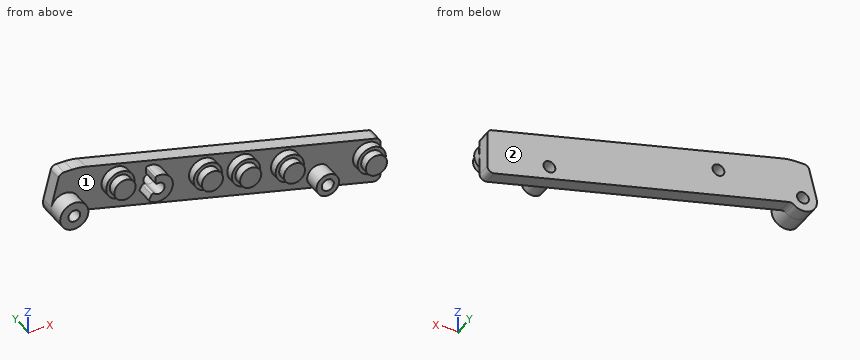
from build123d import *

# Parameters (mm, degrees)
SKETCH1_R           = 2.667
BOSS_EXTRUDE1_DEPTH = 6.35
SKETCH3_R           = 6.35
BOSS_EXTRUDE2_DEPTH = 3.81
SKETCH4_R           = 4.7625
BOSS_EXTRUDE3_DEPTH = 3.81
SKETCH5_R           = 6.35
SKETCH5_R_2         = 2.667
SKETCH5_R_3         = 5.08
SKETCH5_R_4         = 2.723974981
BOSS_EXTRUDE4_DEPTH = 7.62


with BuildPart() as part:
    # Sketch1 → Boss-Extrude1 (new body)
    with BuildSketch(Plane(origin=(0, 0, 0), x_dir=(-1, 0, 0), z_dir=(0, 1, 0))):
        with BuildLine():
            Line((132.859114436, 54.06756661), (1.925518385, 21.422154602))
            ThreePointArc((1.925518385, 21.422154602), (0.538452686, 20.521383604), (0, 18.957603457))
            Line((0, 18.957603457), (0, 3.251051746))
            ThreePointArc((0, 3.251051746), (0.976219853, 1.249504432), (3.154481615, 0.786500601))
            Line((3.154481615, 0.786500601), (135.868185597, 33.875743365))
            ThreePointArc((135.868185597, 33.875743365), (137.061865325, 33.884273202), (138.127619437, 33.346581632))
            ThreePointArc((138.127619437, 33.346581632), (145.587943549, 32.789337046), (148.401377862, 39.7212592))
            Line((148.401377862, 39.7212592), (145.116412217, 52.896536778))
            ThreePointArc((145.116412217, 52.896536778), (144.215641219, 54.283602477), (142.651861072, 54.822055163))
            Line((142.651861072, 54.822055163), (139.003930584, 54.822055163))
            ThreePointArc((139.003930584, 54.822055163), (135.908449262, 54.632727414), (132.859114436, 54.06756661))
        make_face()
        with Locations(Location((142.24, 38.185055163, 0), (0, 0, 90))):
            Circle(SKETCH1_R, mode=Mode.SUBTRACT)
        with Locations(Location((27.94, 12.785055202, 0), (0, 0, 90))):
            Circle(SKETCH1_R, mode=Mode.SUBTRACT)
        with Locations(Location((104.14, 38.185055202, 0), (0, 0, 90))):
            Circle(SKETCH1_R, mode=Mode.SUBTRACT)
    extrude(amount=-BOSS_EXTRUDE1_DEPTH)

    # Sketch3 → Boss-Extrude2 (add)
    with BuildSketch(Plane(origin=(0, -6.35, 0), x_dir=(-1, 0, 0), z_dir=(0, -1, 0))):
        with Locations(Location((6.00871488, -14.586933973, 0), (0, 0, 198.870092131))):
            Circle(SKETCH3_R)
        with Locations(Location((42.976982051, -23.804158196, 0), (0, 0, 270))):
            Circle(SKETCH3_R)
        with Locations(Location((79.945249222, -33.021382418, 0), (0, 0, 270))):
            Circle(SKETCH3_R)
        with Locations(Location((119.378067538, -42.853088255, 0), (0, 0, 270))):
            Circle(SKETCH3_R)
        with Locations(Location((62.693391209, -28.720011114, 0), (0, 0, 270))):
            Circle(SKETCH3_R)
    extrude(amount=BOSS_EXTRUDE2_DEPTH)

    # Sketch4 → Boss-Extrude3 (add)
    with BuildSketch(Plane.XZ.offset(10.16)):
        with Locations(Location((-6.00871488, 14.586933973, 0), (0, 0, 90))):
            Circle(SKETCH4_R)
        with Locations(Location((-42.976982051, 23.804158196, 0), (0, 0, 90))):
            Circle(SKETCH4_R)
        with Locations(Location((-62.693391209, 28.720011114, 0), (0, 0, 90))):
            Circle(SKETCH4_R)
        with Locations(Location((-79.945249222, 33.021382418, 0), (0, 0, 90))):
            Circle(SKETCH4_R)
        with Locations(Location((-119.378067538, 42.853088255, 0), (0, 0, 90))):
            Circle(SKETCH4_R)
    extrude(amount=BOSS_EXTRUDE3_DEPTH)

    # Sketch5 → Boss-Extrude4 (add)
    with BuildSketch(Plane.XZ.offset(6.35)):
        with Locations(Location((-142.24, 38.185055163, 0), (0, 0, 166))):
            Circle(SKETCH5_R)
        with Locations(Location((-142.24, 38.185055163, 0), (0, 0, 90))):
            Circle(SKETCH5_R_2, mode=Mode.SUBTRACT)
        with Locations(Location((-27.94, 12.785055202, 0), (0, 0, 270))):
            Circle(SKETCH5_R_3)
        with Locations(Location((-27.94, 12.785055202, 0), (0, 0, 270))):
            Circle(SKETCH5_R_4, mode=Mode.SUBTRACT)
        with BuildLine():
            Line((-105.580163175, 43.777970545), (-105.715311414, 41.562252701))
            ThreePointArc((-105.715311414, 41.562252701), (-105.443232026, 40.931048752), (-104.773674962, 40.775681582))
            ThreePointArc((-104.773674962, 40.775681582), (-101.589970205, 37.403878498), (-106.115998075, 36.393876649))
            ThreePointArc((-106.115998075, 36.393876649), (-106.757692083, 36.64019843), (-107.336634242, 36.269696613))
            Line((-107.336634242, 36.269696613), (-108.465736097, 34.358466745))
            ThreePointArc((-108.465736097, 34.358466745), (-108.561892576, 33.849199875), (-108.310080465, 33.396221428))
            ThreePointArc((-108.310080465, 33.396221428), (-98.068500487, 36.325110669), (-104.912246263, 44.487922463))
            ThreePointArc((-104.912246263, 44.487922463), (-105.374571656, 44.25371306), (-105.580163175, 43.777970545))
        make_face()
    extrude(amount=BOSS_EXTRUDE4_DEPTH)


solid = part.part
Geometry: final body of the model. Coordinates: model frame, mm. Face numbers are marked on the shaded views. Coordinates: 2 decimals unless noted, no trailing zeros. Write each loop counter-clockwise with the first axis right and the second up, starting at its lowest first coordinate (ties: lowest second). Pieces come first, ordered by that corner, then holes. Notation, with made-up numbers: (28.5, 69.5) - (87.5, 69.5) arc R13 cw to (87.5, 94.5) - close; hole circle Ø1 at (-12.5, -34). An arc over 180 degrees is marked (long way). Return JSON: item names as keys, results as strings.
Item 1: Section query D-D (x = -59.5). Output: boundary loops of the cut face in (y, z), and give its area (3 significant figures).
Completed:
{"outline": "(-13.97, 25.19) - (-10.16, 25.19) - (-10.16, 23.23) - (-6.35, 23.23) - (-6.35, 14.84) - (0, 14.84) - (0, 35.78) - (-6.35, 35.78) - (-6.35, 34.21) - (-10.16, 34.21) - (-10.16, 32.25) - (-13.97, 32.25) - close", "area": "202 mm2"}
Item 2: Pull-direction query (X, two-part tool) for the marked faces 1 and 2; classes: +X half, -X half, draft (parallel to the pull), parting line (faces both ways), or undercut.
Completed:
{"face 1": "undercut", "face 2": "draft"}
Item 3: Section query B-B (y = -2). Output: boundary loops of the cut face in (x, z).
Completed:
{"outline": "(-148.4, 39.72) arc R6.35 ccw to (-138.13, 33.35) arc R2.54 cw to (-135.87, 33.88) - (-3.15, 0.79) arc R2.54 ccw to (0, 3.25) - (0, 18.96) arc R2.54 ccw to (-1.93, 21.42) - (-132.86, 54.07) arc R25.4 ccw to (-139, 54.82) - (-142.65, 54.82) arc R2.54 ccw to (-145.12, 52.9) - close; hole circle Ø5.33 at (-142.24, 38.19); hole circle Ø5.33 at (-104.14, 38.19); hole circle Ø5.33 at (-27.94, 12.79)"}
Item 4: Line query: L1, parallel to X at y = -6.75, z = 41; L2, parallel to Z at x = -142.24, y = -9.75; L3, parallel to Y at x = -59, z = 19. Output: solid intervals per line, ascending.
Completed:
{"L1": "x = -147.93 to -136.55, -125.45 to -113.3, -105.52 to -98.45", "L2": "z = 31.84 to 35.52, 40.85 to 44.54", "L3": "y = -6.35 to 0"}
Item 5: Section query C-C (x = -27.94). Output: boundary loops of the cut face in (y, z), and give its area (3 significant figures).
Completed:
{"outline": "(-13.97, 7.71) - (-6.35, 7.71) - (-6.35, 6.97) - (0, 6.97) - (0, 10.12) - (-6.35, 10.12) - (-6.35, 10.06) - (-13.97, 10.06) - close; (-13.97, 15.51) - (-6.35, 15.51) - (-6.35, 15.45) - (0, 15.45) - (0, 27.91) - (-6.35, 27.91) - (-6.35, 17.87) - (-13.97, 17.87) - close", "area": "135 mm2"}
Item 6: Section query A-A (y = -11.75). Count the separate pieces of the cut face and the enclosed holes in it, and give its area (3 significant figures).
Completed:
{"separate pieces": "8", "enclosed holes": "2", "area": "591 mm2"}
Item 7: Pin query (flat end, axial travel): pin 1 Ø2 at (x, y) = (-79, -3.5) entering from +Z; pin 2 Ø1 at (x, y) = (-73.5, -6) entering from -Z; pin 3 Ø5 at (y, z) = (-4, 11.5) entering from +X. Return the tip coordinate at first contact, or that it passes through.
Completed:
{"pin 1": "stops at z = 40.89", "pin 2": "stops at z = 18.2", "pin 3": "stops at x = 0"}
